Work out the finished part from the listing and answer in its coordinate system (mm). A direction names the side the tool comes from. Coordinates: 2 decimals unless noted, no trailing zeros. Write each loop counter-clockwise with the first axis right and the second up, starting at its lowest first coordinate (ties: lowest second). Pieces come first, ordered by that corner, then holes. Notation, with made-up numbers: (48.5, -12) - (79.5, -12) arc R6 cw to (79.5, -4) - close; hole circle Ø1 at (-36.75, 51.5). An arc over 180 degrees is marked (long way). Use one line per item in the form item = value. Start each with the question number.
Item 1: A cutting plane is placed at C-C (y = 2.25). Write down the section's boundary in (x, z).
Item 2: Consider probe 1 along Y at (x, z) = (5.25, 0.1); probe 2 along X at (y, z) = (3.25, 1.45); probe 3 along X at (y, z) = (-1, 1.3). Determine where each line is inside the solid, lowest interval first.
Item 3: A cutting plane is placed at A-A (y = 4). Write down the section's boundary in (x, z), then the cut area to 3 significant figures.
Item 4: Given pin 1 (0.8 mm diameter, centred on y = 1, z = 1, fed in from -X); pin 2 (1.5 mm diameter, centred on x = 5.5, y = -1, fed in from +Z), each flat-ended and moving along its own axis, determine where each tip first touches the part or whether it passes through.
Item 5: A cutting plane is placed at B-B (z = 1.35). Write down the section's boundary in (x, y).
Item 6: A cutting plane is placed at D-D (x = 8). Write down the section's boundary in (y, z).
Item 7: Determine the mould class of faces 4 (the flat face through (2.877, 0.919, 0.789)), 5 (the flat face through (5, -6.2, 1)), 6 (the cylindrical face through (-0.315, -0.501, 0.789)), 7 (the flat face through (0.4, 1, 1)) for opening direction Y: released by +Y, released by -Y, zero draft, split by the parting line, or undercut.
Item 8: For faces 1 (the flat face through (9.6, 1, 1)), 2 (the cylindrical face through (9.459, -4.997, 0.789)), 3 (the cylindrical face through (2.177, 5.137, 0.811)), determine the directions among +Z, -Z, +X, -X, +Y, -Y from which every point of the face is accessible in a straight line to the end or side of a thin tool.
Autodesk Inventor part; units mm, degrees
ref_plane "Work Plane1" through (0.2, -0.2, 2) normal (0, 0, -1) x (0, 1, 0)
ref_plane "YZ Plane" through (0, 0, 0) normal (1, 0, 0) x (0, 1, 0)
ref_plane "XZ Plane" through (0, 0, 0) normal (0, 1, 0) x (-1, 0, 0)
sketch "clip_sketch" plane through (0, 0, 0) normal (0, 0, 1) x (1, 0, 0)
  line L0 (0.2, -0.2) -> (9.8, -0.2)
  line L1 (9.8, -0.2) -> (9.8, 2.4)
  line L2 (0.2, 2.4) -> (9.8, 2.4)
  line L3 (0.2, -0.2) -> (0.2, 2.4)
  line L4 (0.4, -0.2) -> (0.4, 2.4)
  line L5 (9.6, 2.4) -> (9.6, -0.2)
  line L6 (0.4, -0.2) -> (0.4, -0.2)
  line L7 (-0.6, -1.2) -> (-0.6, -2.2)
  line L8 (3.4, -6.2) -> (6.6, -6.2)
  line L9 (10.6, -2.2) -> (10.6, -1.2)
  line L10 (9.6, -0.2) -> (9.6, -0.2)
  line L11 (0.4, 2.4) -> (0.4, 5.4)
  line L12 (0.4, 5.4) -> (9.6, 5.4)
  line L13 (9.6, 5.4) -> (9.6, 2.4)
  line L14 (3.4, -4) -> (2.4, 5.4)
  line L15 (6.6, -4) -> (7.6, 5.4)
  arc A0 (0.4, 5.4) -> (0.4, 2.4) centre (2.8, 3.9) ccw
  arc A1 (9.6, 2.4) -> (9.6, 5.4) centre (7.2, 3.9) ccw
  line L16 (5, 2.4) -> (5, -0.2) construction
  arc A2 (0.4, -0.2) -> (-0.6, -1.2) centre (0.4, -1.2) ccw
  arc A3 (10.6, -1.2) -> (9.6, -0.2) centre (9.6, -1.2) ccw
  arc A4 (-0.6, -2.2) -> (3.4, -6.2) centre (3.4, -2.2) ccw
  arc A5 (6.6, -6.2) -> (10.6, -2.2) centre (6.6, -2.2) ccw
  line L17 (3.4, -4) -> (6.6, -4)
  point P0 (0, 0)
  point P1 (-0.6, -0.2)
  dimension "d31" = 0.2
  dimension "d32" = 0.2
  dimension "d33" = 1
  dimension "d34" = 1
  dimension "d35" = 6
  dimension "d36" = 2
  dimension "d37" = 2
  dimension "d39" = 4.4
  dimension "d40" = 4.4
  dimension "d41" = 3
  dimension "d42" = 1
  dimension "d43" = 4
  dimension "d44" = 2.2
  dimension "d45" = 1
ref_plane "Work Plane1" through (0.2, -0.2, 2) normal (0, 0, -1) x (0, 1, 0)
extrude "clip" add sketch "clip_sketch" along normal blind 1.6 contours L4 L2 L14 L0 | L0 L14 L17 L15 A3 L9 A5 L8 A4 L7 A2 | L11 L12 L14 L2 | A0 L11 | L15 L2 L5 L0 | L15 L12 L13 L2 | L13 A1
fillet "teeth" radius 1 4 edges at (2.4, 5.4, 0.8) (7.6, 5.4, 0.8) (0.4, 5.4, 0.8) (9.6, 5.4, 0.8)
fillet "inside" radius 1.6 2 edges at (3.4, -4, 0.8) (6.6, -4, 0.8)
properties part number "fastener_lock" material "ABS Plastic"
Answer:
q1.outline = (0.4, 0) - (2.74, 0) - (2.74, 1.6) - (0.4, 1.6) - close; (7.26, 0) - (9.6, 0) - (9.6, 1.6) - (7.26, 1.6) - close
q2.probe_1 = -6.2 to -4
q2.probe_2 = 0.05 to 2.63, 7.37 to 9.95
q2.probe_3 = -0.58 to 3.08, 6.92 to 10.58
q3.outline = (-0.03, 0) - (2.55, 0) - (2.55, 1.6) - (-0.03, 1.6) - close; (7.45, 0) - (10.03, 0) - (10.03, 1.6) - (7.45, 1.6) - close
q3.area = 8.25 mm²
q4.pin_1 = 0.4
q4.pin_2 = through
q5.outline = (-0.6, -2.2) arc R4 ccw to (3.4, -6.2) - (6.6, -6.2) arc R4 ccw to (10.6, -2.2) - (10.6, -1.2) arc R1 ccw to (9.6, -0.2) - (9.6, 2.4) arc R2.83 ccw to (9.92, 4.67) arc R1 ccw to (8.96, 5.4) - (8.5, 5.4) arc R1 ccw to (7.5, 4.51) - (6.75, -2.57) arc R1.6 cw to (5.16, -4) - (4.84, -4) arc R1.6 cw to (3.25, -2.57) - (2.5, 4.51) arc R1 ccw to (1.5, 5.4) - (1.04, 5.4) arc R1 ccw to (0.08, 4.67) arc R2.83 ccw to (0.4, 2.4) - (0.4, -0.2) arc R1 ccw to (-0.6, -1.2) - close
q6.outline = (-5.95, 0) - (5.27, 0) - (5.27, 1.6) - (-5.95, 1.6) - close
q7.face_4 = released by +Y
q7.face_5 = released by -Y
q7.face_6 = undercut
q7.face_7 = undercut
q8.face_1 = +Z, -Z, +X
q8.face_2 = +Z, -Z, +X, -Y
q8.face_3 = +Z, -Z, +Y
